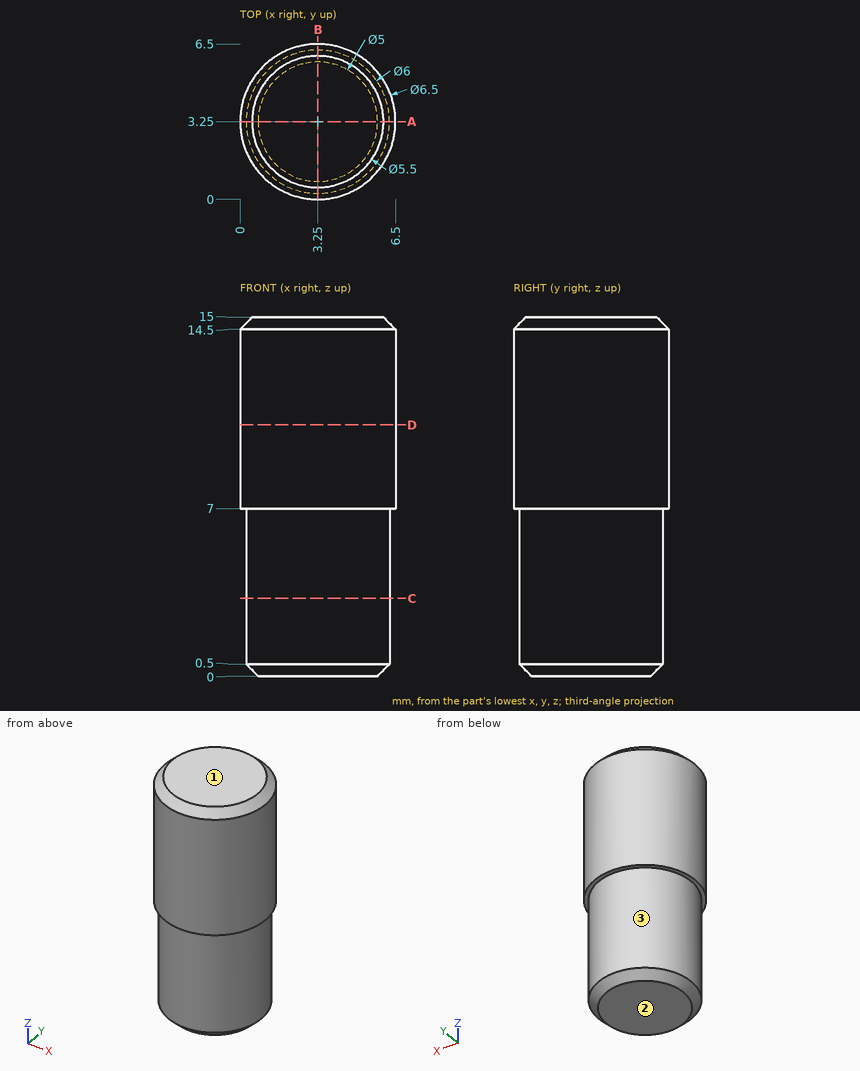
Here's the drawing with two shaded views (mm, measured from the low corner). I have some questions. Give positions to 0.01 mm unless a question says otherwise; leave off trailing zeros. Loops run counter-clockwise (first coordinate to the right, second up) from the corner with the lowest first, then second, coordinate; pieces in that order, holes last. Notation, with made-up numbers: (67.5, -17.5) -> (109.5, -17.5) arc R30 cw to (109.5, 21.5) -> close; hole circle Ø3 at (31.25, 77.5). An arc over 180 degrees is marked (long way). Use one line per item in the form item = value.
1) If we section it at A-A (y = 3.25): Please give me the cut outline in (x, z), plus the area to 3 significant figures.
Answers:
outline = (0, 7) -> (0.25, 7) -> (0.25, 0.5) -> (0.75, 0) -> (5.75, 0) -> (6.25, 0.5) -> (6.25, 7) -> (6.5, 7) -> (6.5, 14.5) -> (6, 15) -> (0.5, 15) -> (0, 14.5) -> close
area = 93.5 mm²
2) We'd pull the mould along Z, two halves only. Please class the marked faces 1, 2 and 3: released by +Z, released by -Z, zero draft, split by the parting line, or undercut.
Answers:
face_1 = released by +Z
face_2 = released by -Z
face_3 = zero draft
3) If we section it at D-D (z = 10.5): Please give me the cut outline in (x, y).
Answers:
outline = circle Ø6.5 at (3.25, 3.25)
4) Will this pin go through, and if not, where does the flat tip stop? pin 1 (1 mm diameter, centred on y = 3, z = 4.5, fed in from +X).
Answers:
pin_1 = 6.25
5) I need wall thicknesses on line 1 along X through (y, z) = (2.75, 12.75); line 2 along Z through (x, y) = (5.5, 4.75); line 3 along Z through (x, y) = (1.5, 1). Which ranges of each line are inside material? Lowest first, please.
Answers:
line_1 = 0.04 to 6.46
line_2 = 0.2 to 15
line_3 = 0.35 to 14.9
6) If we section it at C-C (z = 3.25): Please give me the cut outline in (x, y).
Answers:
outline = circle Ø6 at (3.25, 3.25)
